```python
from build123d import *

# Parameters (mm, degrees)
ESQUISSE1_R        = 3
ESQUISSE1_R_2      = 1.25
BOSS_EXTRU_1_DEPTH = 4
CHANFREIN1_SIZE    = 0.2
CHANFREIN1_SIZE2   = 0.549495484
ESQUISSE2_R        = 2
BOSS_EXTRU_2_DEPTH = 6
ESQUISSE3_R        = 3.75
ESQUISSE3_R_2      = 2
BOSS_EXTRU_3_DEPTH = 8
CONG_3_R           = 0.3
ESQUISSE4_W        = 1.5
ESQUISSE4_H        = 0.5
CONG_4_R           = 0.3
CONG_5_R           = 0.15


with BuildPart() as part:
    # Esquisse1 → Boss.-Extru.1 (new body)
    with BuildSketch(Plane.XY):
        Circle(ESQUISSE1_R)
        Circle(ESQUISSE1_R_2, mode=Mode.SUBTRACT)
    extrude(amount=BOSS_EXTRU_1_DEPTH)

    # Chanfrein1
    chanfrein1_edges = [part.edges().sort_by_distance(p)[0] for p in [
        (-3, 0, 0),
    ]]
    chanfrein1_side = [part.faces().sort_by_distance(p)[0] for p in [
        (-2.915147186, 0, 0),
    ]]
    chamfer(chanfrein1_edges, length=CHANFREIN1_SIZE, length2=CHANFREIN1_SIZE2, reference=chanfrein1_side[0])

    # Esquisse2 → Boss.-Extru.2 (add)
    with BuildSketch(Plane.XY.offset(4)):
        Polygon((2.309401077, -4), (4.618802154, 0), (2.309401077, 4), (-2.309401077, 4), (-4.618802154, 0), (-2.309401077, -4), align=None)
        Circle(ESQUISSE2_R, mode=Mode.SUBTRACT)
    extrude(amount=BOSS_EXTRU_2_DEPTH)

    # Esquisse3 → Boss.-Extru.3 (add)
    with BuildSketch(Plane.XY.offset(10)):
        Circle(ESQUISSE3_R)
        Circle(ESQUISSE3_R_2, mode=Mode.SUBTRACT)
    extrude(amount=BOSS_EXTRU_3_DEPTH)

    # Congé3
    cong_3_edges = [part.edges().sort_by_distance(p)[0] for p in [
        (-3, 0, 4),
    ]]
    fillet(cong_3_edges, radius=CONG_3_R)

    # Esquisse4 → Enlèvement de matière-Révolution1 (revolve, cut)
    with BuildSketch(Plane(origin=(0, 0, 0), x_dir=(1, 0, 0), z_dir=(0, 1, 0))):
        with Locations((3, -16.25)):
            Rectangle(ESQUISSE4_W, ESQUISSE4_H)
    revolve(axis=Axis((0, 0, 52.241443479), (0, 0, -1)), mode=Mode.SUBTRACT)

    # Congé4
    cong_4_edges = [part.edges().sort_by_distance(p)[0] for p in [
        (-3.75, 0, 18),
    ]]
    fillet(cong_4_edges, radius=CONG_4_R)

    # Congé5
    cong_5_edges = [part.edges().sort_by_distance(p)[0] for p in [
        (-3.75, 0, 16),
        (-3.75, 0, 16.5),
    ]]
    fillet(cong_5_edges, radius=CONG_5_R)


solid = part.part
```
Model file for the job. Use its own axes, mm. A direction names the side the tool comes from. Round coordinates to 2 decimals unless told otherwise and drop trailing zeros. Write each loop counter-clockwise with the first axis right and the second up, starting at its lowest first coordinate (ties: lowest second). Pieces come first, ordered by that corner, then holes. Notation, with made-up numbers: (-31.75, 71) - (-20.75, 71) arc R8 cw to (-20.75, 86) - close; hole circle Ø11 at (85, 74). An arc over 180 degrees is marked (long way). Use CSV: the item, a comma, the result in double quotes. Start each with the question number.
Item 1: Tool access for faces 4 (the face through (-0.29, -2.23, 16.25)), 5 (the face through (-3, 0, 2)), 6 (the face through (0, 4, 7)), 7 (the face through (-3.746, 0.165, 17.168)): list every direction of +Z, -Z, +X, -X, +Y, -Y with a clear straight run to the whole face (end or side of a thin tool).
Item 2: Band-saw the part on B-B (z = 2.5). Write the cut outline in (x, y), and give its area (3 significant figures).
Item 3: Band-saw the part on A-A (z = 5). Write the cut outline in (x, y).
Item 4: Pin check, flat tips, straight feed: P1, Ø2, axis at y = 0, z = 10.5, coming from the +X side; P2, Ø4, axis at y = -1, z = 7.5, coming from the -X side; P3, Ø2, axis at x = 0, y = 0, coming from the -Z side. Stop position of each tip, or through.
Item 5: Two-plate mould, pull along Z, no slides. Class faces 1 (the face through (2, 2, 16.5)), 2 (the face through (1, -1, 0)), 3 (the face through (-3.746, 0.165, 12.884)): released by +Z, released by -Z, zero draft, split by the parting line, or undercut.
Item 6: Drill centre lines: L1, parallel to Z at x = -0.5, y = -3.25; L2, parallel to Y at x = 0, z = 2.9; L3, parallel to Y at x = -3, z = 7.25. Where is each one in solid material? Low to high. Write a range as [from, to].
Checked values:
1,face 4,"none"
1,face 5,"-Z"
1,face 6,"+Z, -Z, +X, -X, +Y"
1,face 7,"+Z"
2,outline,"circle Ø6 at (0, 0); hole circle Ø2.5 at (0, 0)"
2,area,"23.4 mm²"
3,outline,"(-4.62, 0) - (-2.31, -4) - (2.31, -4) - (4.62, 0) - (2.31, 4) - (-2.31, 4) - close; hole circle Ø4 at (0, 0)"
4,P1,"stops at x = 4.62"
4,P2,"stops at x = -4.62"
4,P3,"passes through"
5,face 1,"undercut"
5,face 2,"released by -Z"
5,face 3,"zero draft"
6,L1,"z = [4, 16], [16.5, 18]"
6,L2,"y = [-3, -1.25], [1.25, 3]"
6,L3,"y = [-2.8, 2.8]"
